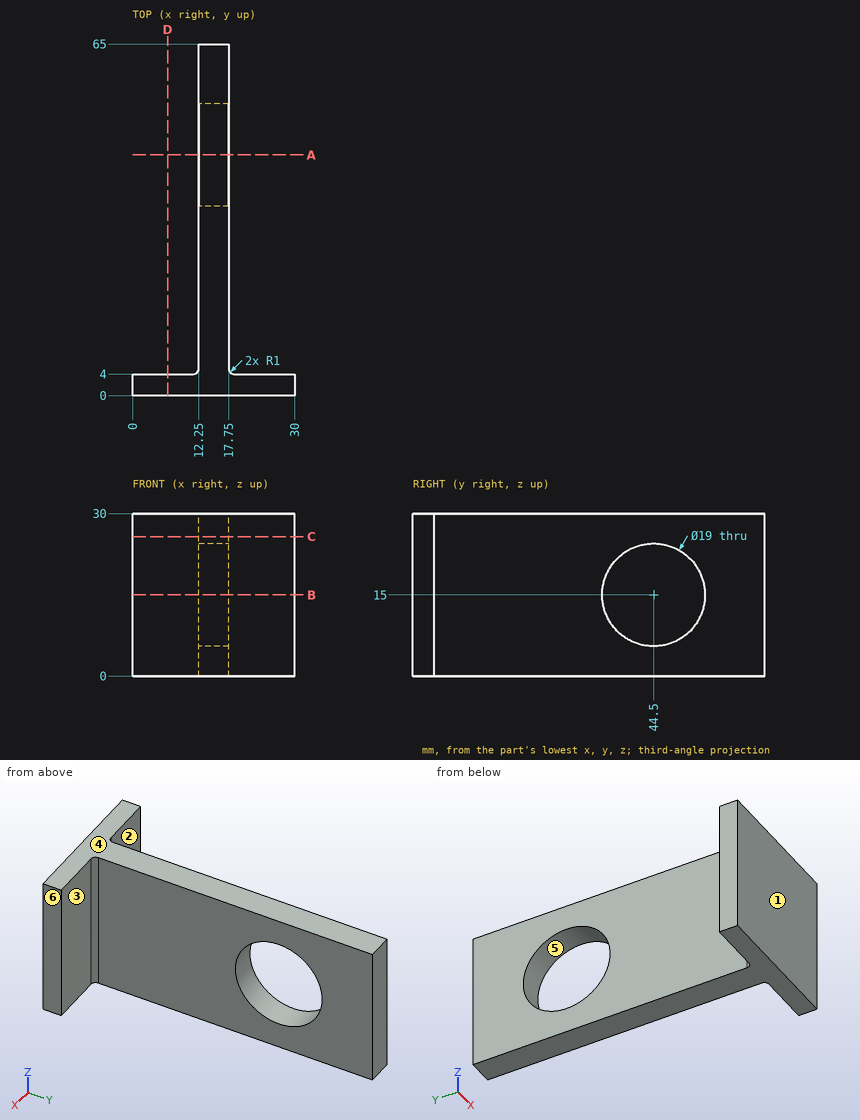
The drawing under review shows one solid part. Ordinate dimensions are in mm from its lowest x, y, z. A direction names the side the tool comes from. Give positions to 0.01 mm unless a question says otherwise; leave off trailing zeros. Write each loop counter-clockwise with the first axis right and the second up, starting at its lowest first coordinate (ties: lowest second). Pieces come first, ordered by that corner, then holes.
1. Add section B-B, the plane z = 15. Write out the cut boundary in (x, y), plus the area to 3 significant figures.
2. For P1, Ø10, axis at x = 8, y = 51, coming from the -Z side; P2, Ø8, axis at y = 21, z = 11, coming from the +X side; P3, Ø15, axis at y = 44.5, z = 15, coming from the +X side; P4, Ø15, axis at y = 41, z = 19.5, coming from the -X side, all flat-tipped, find the tip position at first contact; note any pin that passes through.
3. Draft analysis for pull direction Z (two halves, no side actions). For the marked faces 4, 5 and 6, state which applies: +Z half, -Z half, draft (parallel to the pull), parting line (faces both ways), or undercut.
4. Tool access review of the marked faces 1, 2 and 3: name each direction out of +Z, -Z, +X, -X, +Y, -Y from which nothing blocks a thin tool from reaching the whole face with its end or side.
5. Wall thickness on L1, parallel to Y at x = 16.4, z = 15; L2, parallel to X at y = 24, z = 3.75; L3, parallel to Y at x = 9.75, z = 10.5: over which ranges is each line inside the solid? List them lowest first.
6. Add section C-C, the plane z = 25.75. Write out the cut boundary in (x, y).
7. Add section A-A, the plane y = 44.5. Write out the cut boundary in (x, z).
8. Add section D-D, the plane x = 6.5. Write out the cut boundary in (y, z), plus the area to 3 significant figures.
Worked answers:
1. outline: (0, 0) - (30, 0) - (30, 4) - (18.75, 4) arc R1 cw to (17.75, 5) - (17.75, 35) - (12.25, 35) - (12.25, 5) arc R1 cw to (11.25, 4) - (0, 4) - close; (12.25, 54) - (17.75, 54) - (17.75, 65) - (12.25, 65) - close
1. area: 351 mm2
2. P1: stops at z = 0
2. P2: stops at x = 17.75
2. P3: passes through
2. P4: stops at x = 12.25
3. face 4: +Z half
3. face 5: undercut
3. face 6: draft
4. face 1: +Z, -Z, +X, -X, -Y
4. face 2: +Z, -Z, -X, +Y
4. face 3: +Z, -Z, +X, +Y
5. L1: y = 0 to 35, 54 to 65
5. L2: x = 12.25 to 17.75
5. L3: y = 0 to 4
6. outline: (0, 0) - (30, 0) - (30, 4) - (18.75, 4) arc R1 cw to (17.75, 5) - (17.75, 65) - (12.25, 65) - (12.25, 5) arc R1 cw to (11.25, 4) - (0, 4) - close
7. outline: (12.25, 0) - (17.75, 0) - (17.75, 5.5) - (12.25, 5.5) - close; (12.25, 24.5) - (17.75, 24.5) - (17.75, 30) - (12.25, 30) - close
8. outline: (0, 0) - (4, 0) - (4, 30) - (0, 30) - close
8. area: 120 mm2
